Source: CAD feature listing. Evaluate the final solid. Frame: model axes, mm. Face numbers are marked on the shaded views. Coordinates: 2 decimals unless noted, no trailing zeros. Write each loop counter-clockwise with the first axis right and the second up, starting at its lowest first coordinate (ties: lowest second). Pieces come first, ordered by that corner, then holes. Notation, with made-up numbers: (-22, 67.25) -> (-7, 67.25) arc R9 ccw to (-7, 72.25) -> close; hole circle Ø7 at (30, 31). An arc over 180 degrees is marked (long way). One line per item, written item: value. Start each with the question number.
1. Line query: line 1 (X direction, y = 1.25, z = 4.5); line 2 (X direction, y = 5.5, z = -5.25); line 3 (X direction, y = 3.75, z = -3). Output: solid intervals per line, ascending.
2. Section query C-C, the plane z = 3.25. Output: boundary loops of the cut face in (x, y) (1 decimal), and give its area (3 significant figures).
3. Section query A-A, the plane x = 0. Output: boundary loops of the cut face in (y, z) (3 decimals).
4. Section query B-B, the plane y = 2.75. Output: boundary loops of the cut face in (x, z) (3 decimals), and give its area (3 significant figures).
5. Mould query, pull axis Z, two halves, no side actions, for the marked faces 1, 2 and 3. Classes: released by +Z, released by -Z, zero draft, split by the parting line, or undercut.
6. Section query D-D, the plane y = 9.25. Output: boundary loops of the cut face in (x, z).
7. First-contact query: P1, Ø1.7, axis at x = -2.5, z = 3.5, coming from the +Y side; P2, Ø1.7, axis at y = 0.5, z = 4, coming from the +X side; P3, Ø1.3, axis at y = 0.5, z = 4, coming from the -X side; P4, Ø4, axis at x = -4.5, y = 5.5, coming from the -Z side. Flat tips, straight axial feed; report the tip coordinate or a pass-through.
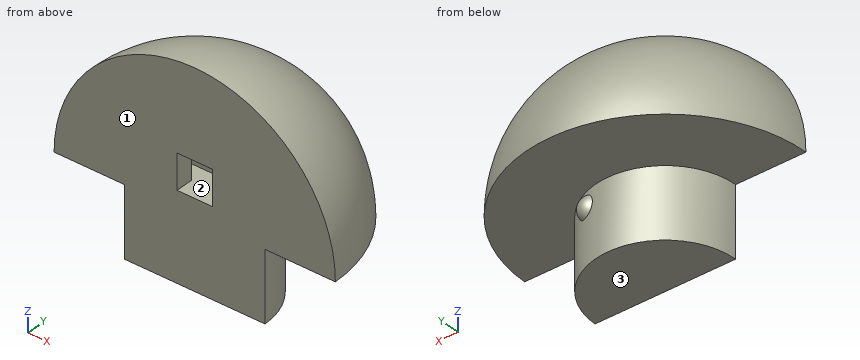
from build123d import *

# Parameters (mm, degrees)
F1_ANGLE = 180
F2_W     = 3.175
F2_H     = 3.175
F3_DEPTH = 3.175
F4_W     = 1.5875
F4_H     = 3.175
F5_DEPTH = 1.5875
F6_W     = 1.5875
F6_H     = 3.175
F7_DEPTH = 1.5875


with BuildPart() as f1:
    # F0 (on Front) → F1 (revolve)
    with BuildSketch(Plane.XZ):
        with BuildLine():
            Line((6.35, 0), (12.7, 0))
            ThreePointArc((12.7, 0), (8.9802561211, 8.9802561211), (0, 12.7))
            Line((0, 12.7), (0, 0))
            Line((0, 0), (0, -6.35))
            Line((0, -6.35), (6.35, -6.35))
            Line((6.35, -6.35), (6.35, 0))
        make_face()
    revolve(axis=Axis((0, 0, 3.175), (0, 0, 1)), revolution_arc=F1_ANGLE)

    # F2 (on face) → F3 (cut)
    with BuildSketch(Plane.XZ):
        with Locations((0, 3.1705502801)):
            Rectangle(F2_W, F2_H)
    extrude(amount=-F3_DEPTH, mode=Mode.SUBTRACT)

    # F4 (on face) → F5 (cut)
    with BuildSketch(Plane(origin=(1.5875, 0, 0), x_dir=(0, -1, 0), z_dir=(-1, 0, 0))):
        with Locations((-2.38125, 3.1705502801)):
            Rectangle(F4_W, F4_H)
    extrude(amount=-F5_DEPTH, mode=Mode.SUBTRACT)

    # F6 (on face) → F7 (cut)
    with BuildSketch(Plane.YZ.offset(-1.5875)):
        with Locations((2.38125, 3.1705502801)):
            Rectangle(F6_W, F6_H)
    extrude(amount=-F7_DEPTH, mode=Mode.SUBTRACT)

    # F10 (on offset) → F11 (revolve)
    with BuildSketch(Plane.XZ.offset(-5.334)):
        with BuildLine():
            Line((2.2999537177, -1.2474206742), (2.2999537177, -0.1679093605))
            ThreePointArc((2.2999537177, -0.1679093605), (1.2204424041, -1.2474206742), (2.2999537177, -2.3269319879))
            Line((2.2999537177, -2.3269319879), (2.2999537177, -1.2474206742))
        make_face()
    revolve(axis=Axis((2.2999537177, 5.334, -1.787176331), (0, 0, -1)))


solid = f1.part
Computed values:
1. line 1: x = -11.81 to -1.59, 1.59 to 11.81
1. line 2: x = -3.17 to 3.17
1. line 3: x = -5.12 to 5.12
2. outline: (-12.3, 0) -> (-1.6, 0) -> (-1.6, 1.6) -> (-3.2, 1.6) -> (-3.2, 3.2) -> (3.2, 3.2) -> (3.2, 1.6) -> (1.6, 1.6) -> (1.6, 0) -> (12.3, 0) arc R12.3 ccw to start
2. area: 222 mm²
3. outline: (0, -6.35) -> (6.35, -6.35) -> (6.35, 0) -> (12.7, 0) arc R12.7 ccw to (0, 12.7) -> (0, 4.758) -> (3.175, 4.758) -> (3.175, 1.583) -> (0, 1.583) -> close
4. outline: (-12.399, 0) -> (-5.724, 0) -> (-5.724, -6.35) -> (5.724, -6.35) -> (5.724, 0) -> (12.399, 0) arc R12.399 ccw to start; hole (-3.175, 1.583) -> (3.175, 1.583) -> (3.175, 4.758) -> (-3.175, 4.758) -> close
4. area: 294 mm²
5. face 1: zero draft
5. face 2: undercut
5. face 3: released by -Z
6. outline: (-8.7, 0) -> (8.7, 0) arc R8.7 ccw to start
7. P1: stops at y = 12.22
7. P2: stops at x = 12.3
7. P3: stops at x = -12.24
7. P4: stops at z = -6.35
